from build123d import *

# Parameters (mm, degrees)
F1_DEPTH = 6.35
F2_W     = 6.35
F2_H     = 228.6
F3_DEPTH = 31.75
F4_R     = 6.35
F5_DEPTH = 762


with BuildPart() as f1:
    # F0 (on Front) → F1 (new body)
    with BuildSketch(Plane.XZ):
        Polygon((-292.1, 114.3), (-330.2, 114.3), (-330.2, -114.3), (-292.1, -114.3), (-285.75, -114.3), (285.75, -114.3), (292.1, -114.3), (330.2, -114.3), (330.2, 114.3), (292.1, 114.3), (285.75, 114.3), (-285.75, 114.3), align=None)
    extrude(amount=F1_DEPTH)

    # F2 (on face) → F3 (join)
    with BuildSketch(Plane.XZ.offset(6.35)):
        with Locations((-288.925, 0)):
            Rectangle(F2_W, F2_H)
        with Locations((288.925, 0)):
            Rectangle(F2_W, F2_H)
        with Locations((-66.675, 0)):
            Rectangle(F2_W, F2_H)
        with Locations((66.675, 0)):
            Rectangle(F2_W, F2_H)
    extrude(amount=F3_DEPTH)

    # F4 (on face) → F5 (cut)
    with BuildSketch(Plane.YZ.offset(292.1)):
        with Locations((-22.225, -88.9)):
            Circle(F4_R)
        with BuildLine():
            Line((-28.575, 88.9), (-28.575, -63.5))
            ThreePointArc((-28.575, -63.5), (-22.092195, -69.848611), (-15.880555, -63.234449))
            Line((-15.880555, -63.234449), (-15.880555, 88.634449))
            Line((-15.880555, 88.634449), (-15.880555, 89.165551))
            ThreePointArc((-15.880555, 89.165551), (-22.357805, 95.248611), (-28.575, 88.9))
        make_face()
        with BuildLine():
            Line((-15.880555, 89.165551), (-15.880555, 88.634449))
            ThreePointArc((-15.880555, 88.634449), (-15.875, 88.9), (-15.880555, 89.165551))
        make_face()
    extrude(amount=-F5_DEPTH, mode=Mode.SUBTRACT)


solid = f1.part
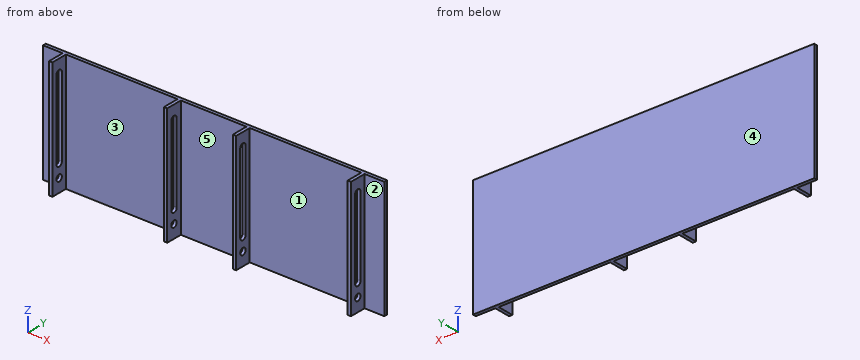
Can you work these out from the model? Positions are in its coordinate system, mm. Face numbers are marked on the shaded views. A direction names the side the tool comes from. Give positions to 0.01 mm unless a question says otherwise; leave off trailing zeros. Order: outer loops, then holes, each group sorted by start corner. A loop starts at its lowest first (then second) coordinate and runs counter-clockwise, first axis right, second up. Notation, with made-up numbers: M -30.5,3 L -16.5,3 A35 ccw -16.5,35 Z; hole C 41,61.5 d10. An arc over 180 degrees is marked long. Use a Markdown table: item, result. Add a question column.
Item 1: We'd pull the mould along X, two halves only. Please class the marked faces 3, 4 and 5: +X half, -X half, draft (parallel to the pull), parting line (faces both ways), or undercut.
Item 2: Will these pins go through, and if not, where does the flat tip stop? pin 1 (19 mm diameter, centred on x = 315, z = -33, fed in from -Y); pin 2 (9.5 mm diameter, centred on y = -26.5, z = 3.5, fed in from -X); pin 3 (10 mm diameter, centred on y = -22.225, z = -88.9, fed in from -X); pin 4 (16.5 mm diameter, centred on y = -22.225, z = -88.9, fed in from +X).
Item 3: If I drill on L1, parallel to X at y = -14, z = -89; L2, parallel to Y at x = -290, z = -88, over which ranges is the centre line in solid material (lowest first)? Write a range as [from, to].
Item 4: For the marked faces 1 and 2, which set-ups out of +Z, -Z, +X, -X, +Y, -Y let a thin tool reach every point of the face, with its end or its side?
Item 5: Suppose I cut it at B-B (x = 36). List the corners of the cut face in (y, z) for me, then the cut area to 3 significant figures.
Item 6: Suppose I cut it at A-A (z = -88.9). Count the separate pieces of the cut face and the enclosed holes in it, then the cut area to 3 significant figures.
Answer sheet:
| question | item | result |
|---|---|---|
| 1 | face 3 | undercut |
| 1 | face 4 | draft |
| 1 | face 5 | undercut |
| 2 | pin 1 | stops at y = -6.35 |
| 2 | pin 2 | stops at x = -292.1 |
| 2 | pin 3 | passes through |
| 2 | pin 4 | stops at x = 292.1 |
| 3 | L1 | x = [-292.1, -285.75], [-69.85, -63.5], [63.5, 69.85], [285.75, 292.1] |
| 3 | L2 | y = [-38.1, -28.51], [-15.94, 0] |
| 4 | face 1 | +Z, -Z, -Y |
| 4 | face 2 | +Z, -Z, +X, -Y |
| 5 | outline | M -6.35,-114.3 L 0,-114.3 L 0,114.3 L -6.35,114.3 Z |
| 5 | area | 1,450 mm² |
| 6 | separate pieces | 5 |
| 6 | enclosed holes | 0 |
| 6 | area | 4,680 mm² |
